from build123d import *

# Parameters (mm, degrees)
EXTRUDE_START       = 3
SKETCH_1_R          = 4.5
EXTRUDE_1_DEPTH     = 12
CUT_EXTRUDE_3_DEPTH = 5
SKETCH_3_R          = 2.5
CUT_EXTRUDE_4_DEPTH = 7


with BuildPart() as part:
    # Эскиз1 → Вытянуть1 (new body)
    with BuildSketch(Plane(origin=(0, 0, 0), x_dir=(1, 0, 0), z_dir=(0, 1, 0)).offset(EXTRUDE_START)):
        with Locations(Location((0, 0, 0), (0, 0, 270))):
            Circle(SKETCH_1_R)
    extrude(amount=EXTRUDE_1_DEPTH)

    # Эскиз2 → Вытянуть3 (cut)
    with BuildSketch(Plane(origin=(0, 15, 0), x_dir=(1, 0, 0), z_dir=(0, 1, 0))):
        with BuildLine():
            Line((-2.547547841, 2.4), (2.547547841, 2.4))
            ThreePointArc((2.547547841, 2.4), (3.5, 0), (2.547547841, -2.4))
            Line((2.547547841, -2.4), (-2.547547841, -2.4))
            ThreePointArc((-2.547547841, -2.4), (-3.5, 0), (-2.547547841, 2.4))
        make_face()
    extrude(amount=-CUT_EXTRUDE_3_DEPTH, mode=Mode.SUBTRACT)

    # Эскиз3 → Вытянуть4 (cut)
    with BuildSketch(Plane.XZ.offset(-3)):
        with Locations(Location((0, 0, 0), (0, 0, 270))):
            Circle(SKETCH_3_R)
    extrude(amount=-CUT_EXTRUDE_4_DEPTH, mode=Mode.SUBTRACT)


solid = part.part
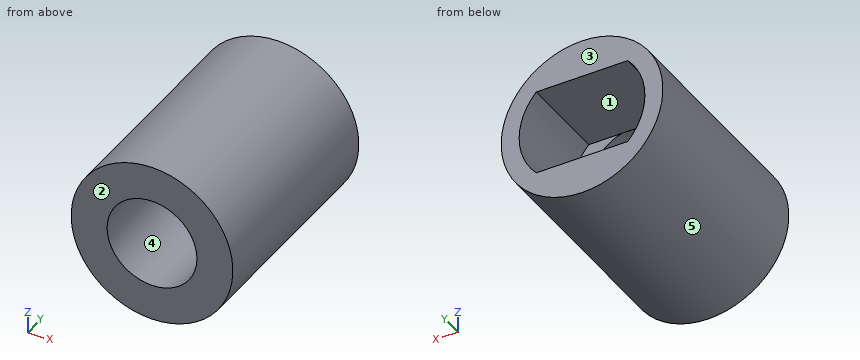
Work out the finished part from the listing and answer in its coordinate system (mm). Face numbers are marked on the shaded views. A direction names the side the tool comes from. Give positions to 0.01 mm unless a question says otherwise; leave off trailing zeros. Order: outer loops, then holes, each group sorted by start corner. A loop starts at its lowest first (then second) coordinate and runs counter-clockwise, first axis right, second up. Notation, with made-up numbers: (-40, 78.5) -> (2, 78.5) arc R14 ccw to (2, 101.5) -> close; hole circle Ø10 at (85.25, 62). An arc over 180 degrees is marked (long way). Answer as a JSON object with one key per item and string values. Group by question number.
1. Section B-B on z = 0 is taken. Determine the outline of the cut face in (x, y).
2. Section D-D on y = 4 is taken. Determine the outline of the cut face in (x, z), plus the area to 3 significant figures.
3. Flat-ended cylindrical pins translate along their axes: pin 1 Ø3 at (x, y) = (-3, 10.5) entering from -Z; pin 2 Ø1.5 at (x, y) = (2.5, 11) entering from +Z; pin 3 Ø4 at (x, y) = (-0.5, 12) entering from -Z; pin 4 Ø2 at (x, z) = (-2, 0) entering from +Y. Find the tip coordinate at first contact, or state that the pin passes through.
4. A tool of negligible diameter and unlimited length cuts with its end or side. For the marked faces 1 and 2, from which of +Z, -Z, +X, -X, +Y, -Y can it reach the whole face along a straight path? Write none if from no direction.
5. The mould has two halves that part along X. Classify the marked faces 3, 4 and 5: released by +X, released by -X, zero draft, split by the parting line, or undercut.
6. Section C-C on y = 13.75 is taken. Determine the outline of the cut face in (x, z).
7. Section A-A on x = 0 is taken. Determine the outline of the cut face in (y, z), plus the area to 3 significant figures.
8. Consider line 1 along X through (y, z) = (5.5, 0); line 2 along X through (y, z) = (7.75, 1.75); line 3 along Z through (x, y) = (-2, 5.25). Determine where each line is inside the solid, lowest interval first. Write a range as [from, to].
Result sheet:
{
 "1": {"outline": "(-4.5, 3) -> (-2.5, 3) -> (-2.5, 10) -> (-3.5, 10) -> (-3.5, 15) -> (-4.5, 15) -> close; (2.5, 3) -> (4.5, 3) -> (4.5, 15) -> (3.5, 15) -> (3.5, 10) -> (2.5, 10) -> close"},
 "2": {"outline": "circle Ø9 at (0, 0); hole circle Ø5 at (0, 0)", "area": "44.0 mm^2"},
 "3": {"pin 1": "stops at z = -4.24", "pin 2": "stops at z = 4.15", "pin 3": "stops at z = -4.5", "pin 4": "stops at y = 10"},
 "4": {"face 1": "+Y", "face 2": "+Z, -Z, +X, -X, -Y"},
 "5": {"face 3": "zero draft", "face 4": "undercut", "face 5": "split by the parting line"},
 "6": {"outline": "circle Ø9 at (0, 0); hole (-2.55, -2.4) -> (2.55, -2.4) arc R3.5 ccw to (2.55, 2.4) -> (-2.55, 2.4) arc R3.5 ccw to start"},
 "7": {"outline": "(3, -4.5) -> (15, -4.5) -> (15, -2.4) -> (10, -2.4) -> (10, -2.5) -> (3, -2.5) -> close; (3, 2.5) -> (10, 2.5) -> (10, 2.4) -> (15, 2.4) -> (15, 4.5) -> (3, 4.5) -> close", "area": "49.0 mm^2"},
 "8": {"line 1": "x = [-4.5, -2.5], [2.5, 4.5]", "line 2": "x = [-4.15, -1.79], [1.79, 4.15]", "line 3": "z = [-4.03, -1.5], [1.5, 4.03]"}
}
